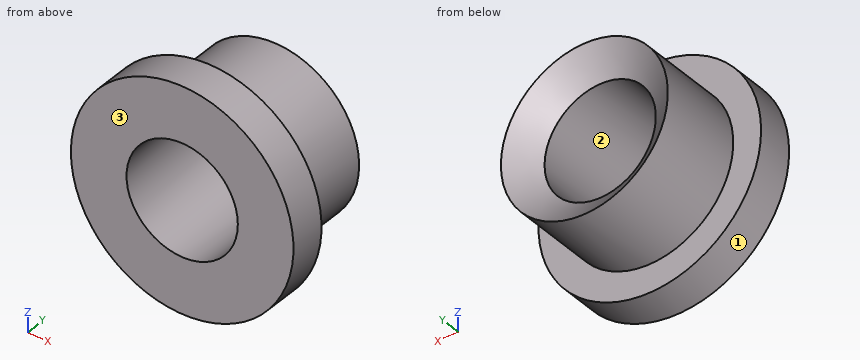
Autodesk Inventor part; units mm, degrees
ref_plane "YZ Plane" through (0, 0, 0) normal (1, 0, 0) x (0, 1, 0)
ref_plane "XZ Plane" through (0, 0, 0) normal (0, 1, 0) x (-1, 0, 0)
ref_plane "XY Plane" through (0, 0, 0) normal (0, 0, 1) x (1, 0, 0)
sketch "Sketch6" plane through (0, 0, 0) normal (0, 1, 0) x (-1, 0, 0)
  circle A0 centre (0, 0) radius 18
  dimension "d30" = 36
extrude "Extrusion4" add sketch "Sketch6" along normal blind 6
sketch "Sketch7" plane through (0, 6, 0) normal (0, 1, 0) x (1, 0, 0)
  circle A0 centre (0, 0) radius 13.5
  dimension "d33" = 27
extrude "Extrusion5" add sketch "Sketch7" along normal blind 14
sketch "Sketch8" plane through (0, 0, 0) normal (0, -1, 0) x (1, 0, 0)
  circle A0 centre (0, 0) radius 9
  dimension "d36" = 18
extrude "Extrusion6" cut sketch "Sketch8" against normal through all
chamfer "Chamfer2" distance 4.5 angle 37 1 edges at (-9, 20, 0) measured on face at (11.7821, 20, 1.7949)
properties part number "00.32.008 \"Bushing\"" material "Steel"
Model file for the job. Use its own axes, mm. Face numbers are marked on the shaded views. Coordinates: 2 decimals unless noted, no trailing zeros. Loops run counter-clockwise (first coordinate to the right, second up) from the corner with the lowest first, then second, coordinate; pieces in that order, holes last. Notation, with made-up numbers: (52, 20) -> (94, 20) arc R26 ccw to (94, 54) -> close; hole circle Ø10 at (23, -2.75). An arc over 180 degrees is marked (long way). Answer as a JSON object with one key per item and string values.
Q1. Pull direction X, two halves, no side cores. Call the marked faces 1, 2 and 3: released by +X, released by -X, zero draft, split by the parting line, or undercut.
Report:
{"face 1": "split by the parting line", "face 2": "undercut", "face 3": "zero draft"}
Q2. Cut at C-C (y = 8). List the corners of the cut face in (x, z).
Report:
{"outline": "circle Ø27 at (0, 0); hole circle Ø18 at (0, 0)"}
Q3. Cut at D-D (y = 2.75). List the corners of the cut face in (x, z), and give its area (3 significant figures).
Report:
{"outline": "circle Ø36 at (0, 0); hole circle Ø18 at (0, 0)", "area": "763 mm2"}
Q4. Flat gauge pins, fed straight in: P1, Ø4, axis at y = 17, z = -1.5, coming from the -X side; P2, Ø1, axis at y = 6, z = 8.5, coming from the +X side; P3, Ø12, axis at y = 14.5, z = 4.5, coming from the +X side. Where does each tip first touch, or does it go through?
Report:
{"P1": "stops at x = -13.5", "P2": "stops at x = 16.12", "P3": "stops at x = 13.5"}
Q5. Probe probe 1 along Z at (x, y) = (0, 9); probe 2 along Y at (x, z) = (-14.5, -0.5); probe 3 along Z at (x, y) = (5, 18.75). List the from-to ranges inside material, lowest first.
Report:
{"probe 1": "z = -13.5 to -9, 9 to 13.5", "probe 2": "y = 0 to 6", "probe 3": "z = -12.54 to -10.73, 10.73 to 12.54"}
